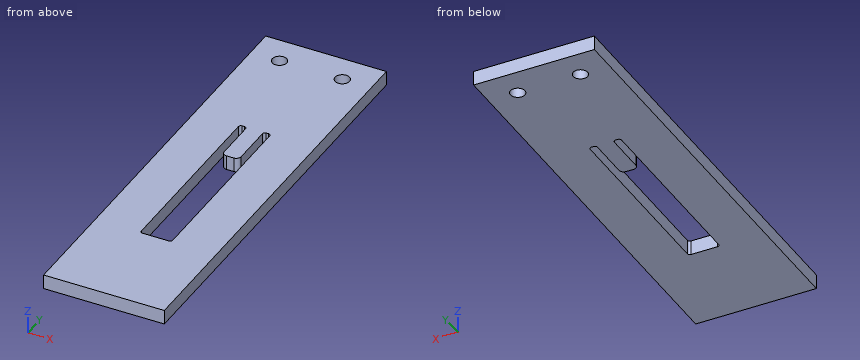
```python
from build123d import *

# Parameters (mm, degrees)
SKETCH1_W           = 25
SKETCH1_H           = 88
BOSS_EXTRUDE1_DEPTH = 3
SKETCH2_R           = 1.5
CUT_EXTRUDE1_DEPTH  = 3
CUT_EXTRUDE2_DEPTH  = 10


with BuildPart() as part:
    # Sketch1 → Boss-Extrude1 (new body)
    with BuildSketch(Plane.XY):
        with Locations((12.5, 44)):
            Rectangle(SKETCH1_W, SKETCH1_H)
    extrude(amount=BOSS_EXTRUDE1_DEPTH)

    # Sketch2 → Cut-Extrude1 (cut)
    with BuildSketch(Plane.XY.offset(3)):
        with Locations((19, 82)):
            Circle(SKETCH2_R)
        with Locations((6, 82)):
            Circle(SKETCH2_R)
    extrude(amount=-CUT_EXTRUDE1_DEPTH, mode=Mode.SUBTRACT)

    # Sketch3 → Cut-Extrude2 (cut)
    with BuildSketch(Plane.XY.offset(3)):
        with BuildLine():
            Line((9.75, 20.5), (15.25, 20.5))
            ThreePointArc((15.25, 20.5), (15.603553391, 20.646446609), (15.75, 21))
            Line((15.75, 21), (15.75, 59.5))
            ThreePointArc((15.75, 59.5), (15.603553391, 59.853553391), (15.25, 60))
            Line((15.25, 60), (14.75, 60))
            ThreePointArc((14.75, 60), (14.396446609, 59.853553391), (14.25, 59.5))
            Line((14.25, 59.5), (14.25, 51))
            ThreePointArc((14.25, 51), (13.957106781, 50.292893219), (13.25, 50))
            Line((13.25, 50), (11.75, 50))
            ThreePointArc((11.75, 50), (11.042893219, 50.292893219), (10.75, 51))
            Line((10.75, 51), (10.75, 59.5))
            ThreePointArc((10.75, 59.5), (10.603553391, 59.853553391), (10.25, 60))
            Line((10.25, 60), (9.75, 60))
            ThreePointArc((9.75, 60), (9.396446609, 59.853553391), (9.25, 59.5))
            Line((9.25, 59.5), (9.25, 21))
            ThreePointArc((9.25, 21), (9.396446609, 20.646446609), (9.75, 20.5))
        make_face()
    extrude(amount=-CUT_EXTRUDE2_DEPTH, mode=Mode.SUBTRACT)


solid = part.part
```
Part model, mm, in its own coordinate system. Round coordinates to 2 decimals unless told otherwise and drop trailing zeros. Order: outer loops, then holes, each group sorted by start corner. A loop starts at its lowest first (then second) coordinate and runs counter-clockwise, first axis right, second up. Notation, with made-up numbers: M -11,-13 L -3,-13 A34 cw -3,18 Z; hole C -23,-31.5 d4. An arc over 180 degrees is marked long. Answer in a Markdown table with one row per item. Add a question column.
Q1. Wall check: L1, parallel to X at y = 82, z = 1.6; L2, parallel to Y at x = 19, z = 1.8; L3, parallel to X at y = 26, z = 2. Give the ranges that are in metal, low to high. Write a range as from..to.
Q2. Pin check, flat tip, straight feed: pin 1 (2.5 mm diameter, centred on x = 19, y = 82, fed in from +Z). Stop position of the tip, or through.
Q3. Cut at A-A on y = 82. Give the cut face in (x, z), and give its area (3 significant figures).
Q4. Cut at C-C on z = 0.65. Give the cut face in (x, y).
Q5. Cut at D-D on y = 58. Give the cut face in (x, z).
Q6. Cut at B-B on x = 6. Give the cut face in (y, z), and give its area (3 significant figures).
Established:
| question | item | result |
|---|---|---|
| 1 | L1 | x = 0..4.5, 7.5..17.5, 20.5..25 |
| 1 | L2 | y = 0..80.5, 83.5..88 |
| 1 | L3 | x = 0..9.25, 15.75..25 |
| 2 | pin 1 | passes through |
| 3 | outline | M 0,0 L 4.5,0 L 4.5,3 L 0,3 Z; M 7.5,0 L 17.5,0 L 17.5,3 L 7.5,3 Z; M 20.5,0 L 25,0 L 25,3 L 20.5,3 Z |
| 3 | area | 57.0 mm2 |
| 4 | outline | M 0,0 L 25,0 L 25,88 L 0,88 Z; hole C 6,82 d3; hole M 9.25,21 A0.5 ccw 9.75,20.5 L 15.25,20.5 A0.5 ccw 15.75,21 L 15.75,59.5 A0.5 ccw 15.25,60 L 14.75,60 A0.5 ccw 14.25,59.5 L 14.25,51 A1 cw 13.25,50 L 11.75,50 A1 cw 10.75,51 L 10.75,59.5 A0.5 ccw 10.25,60 L 9.75,60 A0.5 ccw 9.25,59.5 Z; hole C 19,82 d3 |
| 5 | outline | M 0,0 L 9.25,0 L 9.25,3 L 0,3 Z; M 10.75,0 L 14.25,0 L 14.25,3 L 10.75,3 Z; M 15.75,0 L 25,0 L 25,3 L 15.75,3 Z |
| 6 | outline | M 0,0 L 80.5,0 L 80.5,3 L 0,3 Z; M 83.5,0 L 88,0 L 88,3 L 83.5,3 Z |
| 6 | area | 255 mm2 |
